Autodesk Fusion 360 part; units mm, degrees
sketch "Esquisse1" plane through (0, 0, 0) normal (0, 0, 1) x (1, 0, 0)
  line L0 (0, 0) -> (66, 0) construction
  line L1 (66, 53) -> (0, 53) construction
  line L2 (0, 53) -> (0, 0) construction
  line L3 (66, 0) -> (66, 2) construction
  line L4 (66, 2) -> (69, 5) construction
  line L5 (69, 5) -> (69, 37) construction
  line L6 (69, 37) -> (66, 40) construction
  line L7 (66, 40) -> (66, 53) construction
  line L8 (-0.2, -0.2) -> (66.2, -0.2)
  line L9 (66.2, -0.2) -> (66.2, 1.9172)
  line L10 (66.2, 1.9172) -> (69.2, 4.9172)
  line L11 (69.2, 4.9172) -> (69.2, 37.0828)
  line L12 (69.2, 37.0828) -> (66.2, 40.0828)
  line L13 (66.2, 40.0828) -> (66.2, 53.2)
  line L14 (66.2, 53.2) -> (-0.2, 53.2)
  line L15 (-0.2, 53.2) -> (-0.2, -0.2)
  dimension "d1" = 66
  dimension "d2" = 53
  dimension "d6" = 37
  dimension "d7" = 40
  dimension "d10" = 3
  dimension "d11" = 3
  dimension "d12" = 2
  dimension "d24" = 0.2
sketch "Esquisse2" plane through (0, 0, 0) normal (0, 0, 1) x (1, 0, 0)
  circle A0 centre (14.1, 2.5) radius 1
  circle A1 centre (66.5, 35) radius 1
  circle A2 centre (66.5, 7) radius 1
  line L0 (0, 53) -> (0, 0)
  line L1 (66, 53) -> (0, 53)
  line L2 (69, 5) -> (69, 37)
  line L3 (66.5, 7) -> (66.5, 35) construction
  line L4 (0, 0) -> (66, 0) construction
  circle A3 centre (14.1, 2.5) radius 2.7
  circle A4 centre (66.5, 35) radius 2.7
  circle A5 centre (66.5, 7) radius 2.7
  line L5 (69.2, 37.0828) -> (66.2, 40.0828)
  line L6 (66.2, 40.0828) -> (66.2, 53.2)
  line L7 (66.2, 40.0828) -> (64.1305, 36.2944)
  line L8 (69.2, 4.9172) -> (69.2, 37.0828)
  line L9 (66.5, 32.3) -> (69.2, 32.3)
  arc A6 (64.1305, 36.2944) -> (66.5, 32.3) centre (66.5, 35) ccw
  line L10 (66.2, 1.9172) -> (69.2, 4.9172)
  line L11 (66.2, -0.2) -> (66.2, 1.9172)
  line L12 (66.2, 1.9172) -> (64.1305, 5.7056)
  line L13 (66.5, 9.7) -> (69.2, 9.7)
  arc A7 (66.5, 9.7) -> (64.1305, 5.7056) centre (66.5, 7) ccw
  line L14 (-0.2, -0.2) -> (66.2, -0.2)
  line L15 (16.8, 2.5) -> (16.8, -0.2)
  line L16 (11.4, 2.5) -> (11.4, -0.2)
  arc A8 (16.8, 2.5) -> (11.4, 2.5) centre (14.1, 2.5) ccw
  line L17 (0, 48) -> (10, 48)
  line L18 (10, 48) -> (10, 53) construction
  arc A9 (10, 48) -> (15, 53) centre (10, 53) ccw
  dimension "d14" = 2
  dimension "d15" = 2
  dimension "d16" = 2
  dimension "d17" = 14.1
  dimension "d20" = 2.5
  dimension "d21" = 7
  dimension "d22" = 2
  dimension "d33" = 1.7
  dimension "d34" = 2.5
  dimension "d45" = 5
  dimension "d46" = 10
  dimension "d85" = 2.7
sketch "Esquisse3" plane through (0, 0, 0) normal (0, 0, 1) x (1, 0, 0)
  line L0 (-4, -1.7) -> (70.7, -1.7)
  line L1 (70.7, -1.7) -> (70.7, 54.7)
  line L2 (70.7, 54.7) -> (-4, 54.7)
  line L3 (-4, 54.7) -> (-4, -1.7)
  line L4 (-0.2, -0.2) -> (66.2, -0.2)
  line L5 (69.2, 4.9172) -> (69.2, 37.0828)
  line L6 (-5, -2.7) -> (71.7, -2.7)
  line L7 (71.7, -2.7) -> (71.7, 55.7)
  line L8 (71.7, 55.7) -> (-5, 55.7)
  line L9 (-5, 55.7) -> (-5, -2.7)
  dimension "d26" = 56.4
  dimension "d27" = 1.5
  dimension "d28" = 74.7
  dimension "d29" = 1.5
  dimension "d52" = 1
extrude "Extrusion1" add sketch "Esquisse3" against normal blind 1.5 contours L0 L1 L2 L3
sketch "Esquisse4" plane through (0, 0, 0) normal (0, 0, 1) x (-1, 0, 0)
  line L0 (4, -54.7) -> (4, 1.7)
  line L1 (4, 1.7) -> (-70.7, 1.7)
  line L2 (-70.7, 1.7) -> (-70.7, -54.7)
  line L3 (-70.7, -54.7) -> (4, -54.7)
  line L4 (4, -54.7) -> (-70.7, -54.7)
  line L5 (-70.7, -54.7) -> (-70.7, 1.7)
  line L6 (-70.7, 1.7) -> (4, 1.7)
  line L7 (4, 1.7) -> (4, -54.7)
  line L8 (2.5, -53.2) -> (-69.2, -53.2)
  line L9 (-69.2, -53.2) -> (-69.2, 0.2)
  line L10 (-69.2, 0.2) -> (2.5, 0.2)
  line L11 (2.5, 0.2) -> (2.5, -53.2)
  line L12 (-66.2, 0.2) -> (-66.2, -1.9172)
  line L13 (-66.2, -1.9172) -> (-69.2, -4.9172)
  line L14 (-66.2, -40.0828) -> (-66.2, -53.2)
  line L15 (-69.2, -37.0828) -> (-66.2, -40.0828)
  line L16 (0.2, -53.2) -> (0.2, 0.2)
  dimension "d32" = 1.5
extrude "Extrusion2" add sketch "Esquisse2" along normal blind 2 contours L2 A5 A7 | L2 A4 A6 | A3 A8
extrude "Extrusion3" cut 3 faces at (16.2233, 2.6341, 2) (68.5, 7, 2) (68.5, 35, 2) along direction (0, 0, -1) blind 2
extrude "Extrusion4" add sketch "Esquisse2" sketch "Esquisse4" along normal blind 3 contours L2 A5 A7 | A5 L8 L10 L12 | L2 A5 | L2 A5 L13 | L2 A5 L8 L13 | A3 L14 L15 | L2 A4 L9 | L2 A4 L8 L9 | L2 A4 A6 | L2 A4 | A4 L5 L7 L8 | A3 L14 L16 | A3 A8 of sketch 2 contours L8 L9 L14 L15 | L9 L10 L12 L13
extrude "Extrusion5" add sketch "Esquisse4" along normal blind 4.5 contours L8 L10 L11 L16
extrude "Extrusion6" add sketch "Esquisse3" sketch "Esquisse4" along normal blind 20.4 and the other way up to surface of sketch 2 second end surface through (0, 0, -1.5) normal (0, 0, -1) offset 0
extrude "Extrusion7" add sketch "Esquisse2" along normal blind 3 contours L0 L1 L17 A9
sketch "Esquisse5" plane through (0, 0, -1.5) normal (0, 0, -1) x (1, 0, 0)
  line L0 (70.7, -26.5) -> (-4, -26.5) construction
  circle A0 centre (45.8, -26.5) radius 1.5
  circle A1 centre (20.9, -26.5) radius 1.5
  line L1 (20.9, -28) -> (-4, -28) construction
  line L2 (20.9, -28) -> (45.8, -28) construction
  line L3 (45.8, -28) -> (70.7, -28) construction
  line L4 (71.7, 2.7) -> (-5, 2.7)
  line L5 (-5, 2.7) -> (-5, -55.7)
  line L6 (-5, -55.7) -> (71.7, -55.7)
  line L7 (71.7, -55.7) -> (71.7, 2.7)
  dimension "d49" = 3
extrude "Extrusion8" cut sketch "Esquisse5" against normal blind 1.5 contours A0 | A1
extrude "Extrusion11" add 1 faces at (-2.5, 17.6, 9.8) along direction (1, 0, 0) blind 1
extrude "Extrusion12" cut 1 faces at (-5, 36.2333, 5.8) along direction (1, 0, 0) blind 1
sketch "Esquisse10" plane through (-1.5, 0, 0) normal (1, 0, 0) x (0, 1, 0)
  line L0 (-0.2, 4.5) -> (53.2, 4.5)
  line L1 (53.2, 4.5) -> (53.2, 20.4)
  line L2 (53.2, 20.4) -> (-0.2, 20.4)
  line L3 (-0.2, 20.4) -> (-0.2, 4.5)
  line L4 (-1.2, 18.9) -> (54.2, 18.9)
  line L5 (54.2, 18.9) -> (54.2, 15.7)
  line L6 (54.2, 15.7) -> (-1.2, 15.7)
  line L7 (-1.2, 15.7) -> (-1.2, 18.9)
  line L8 (26.5, 18.9) -> (26.5, 20.4) construction
  line L9 (-0.2, 18.9) -> (-0.2, 20.4)
  line L10 (-0.2, 20.4) -> (53.2, 20.4)
  dimension "d89" = 1.5
  dimension "d90" = 3.2
  dimension "d93" = 55.4
extrude "Extrusion17" cut sketch "Esquisse10" against normal up to surface (2.5 mm away) contours L3 L4 L6 L7 | L1 L3 L4 L6 | L1 L4 L5 L6 | L1 L2 L3 L4 L9 L10
extrude "Extrusion18" cut sketch "Esquisse10" along normal blind 71.5 contours L3 L4 L6 L7 | L1 L3 L4 L6 | L1 L4 L5 L6
sketch "Esquisse11" plane through (0, 0, 15.7) normal (0, 0, 1) x (-1, 0, 0)
  line L0 (-70, -54.2) -> (4, -54.2)
  line L1 (4, -54.2) -> (4, 1.2)
  line L2 (4, 1.2) -> (-70, 1.2)
  line L3 (-70, 1.2) -> (-70, -54.2)
  line L4 (1.5, -53.2) -> (-69.2, -53.2)
  line L5 (-69.2, -53.2) -> (-69.2, 0.2)
  line L6 (-69.2, 0.2) -> (1.5, 0.2)
  line L7 (1.5, 0.2) -> (1.5, -53.2)
  line L8 (1.9, -54.2) -> (1.9, 1.2)
  dimension "d98" = 71.9
extrude "Extrusion19" add sketch "Esquisse11" along normal blind 0.2 contours L0 L1 L2 L8
sketch "Esquisse7" plane through (-1.5, 0, 0) normal (1, 0, 0) x (0, 1, 0)
  line L0 (-0.2, 15.7) -> (-0.2, 4.5)
  line L1 (-0.2, 4.5) -> (53.2, 4.5)
  line L2 (53.2, 4.5) -> (53.2, 15.7)
  line L3 (3.8, 4.5) -> (13.2, 4.5)
  line L4 (13.2, 4.5) -> (13.2, 15.9)
  line L5 (13.2, 15.9) -> (3.8, 15.9)
  line L6 (3.8, 15.9) -> (3.8, 4.5)
  line L7 (33.4, 4.5) -> (41.8, 4.5)
  line L8 (41.8, 4.5) -> (41.8, 7.7)
  line L9 (41.8, 7.7) -> (33.4, 7.7)
  line L10 (33.4, 7.7) -> (33.4, 4.5)
  line L11 (53.2, 15.7) -> (-0.2, 15.7)
  dimension "d66" = 9.4
  dimension "d67" = 11.4
  dimension "d68" = 4
  dimension "d71" = 8.4
  dimension "d72" = 3.2
  dimension "d73" = 11.4
extrude "Extrusion14" cut sketch "Esquisse7" against normal blind 2.5 contours L1 L3 L4 L6 L11 | L4 L5 L6 L11 | L1 L7 L8 L9 L10
sketch "Esquisse8" plane through (-4, 0, 0) normal (-1, 0, 0) x (0, -1, 0)
  line L0 (-3.8, 4.5) -> (-13.2, 4.5)
  line L1 (-13.2, 4.5) -> (-13.2, 15.9)
  line L2 (-3.8, 15.9) -> (-3.8, 4.5)
  line L3 (-33.4, 4.5) -> (-41.8, 4.5)
  line L4 (-41.8, 4.5) -> (-41.8, 7.7)
  line L5 (-41.8, 7.7) -> (-33.4, 7.7)
  line L6 (-33.4, 7.7) -> (-33.4, 4.5)
  line L7 (-53.2, 20.4) -> (-55.7, 20.4)
  line L8 (-55.7, -1.5) -> (2.7, -1.5)
  line L9 (-31.9, 3) -> (-43.3, 3)
  line L10 (-43.3, 3) -> (-43.3, 9.2)
  line L11 (-43.3, 9.2) -> (-31.9, 9.2)
  line L12 (-31.9, 9.2) -> (-31.9, 3)
  line L13 (2.7, -1.5) -> (2.7, 20.4)
  line L14 (-55.7, 20.4) -> (-55.7, -1.5)
  line L15 (-13.2, 15.9) -> (-54.2, 15.9)
  line L16 (-54.2, 15.9) -> (-54.2, 18.9)
  line L17 (-54.2, 18.9) -> (-53.2, 18.9)
  line L18 (-53.2, 18.9) -> (-53.2, 20.4)
  line L19 (2.7, 20.4) -> (0.2, 20.4)
  line L20 (0.2, 20.4) -> (0.2, 18.9)
  line L21 (0.2, 18.9) -> (1.2, 18.9)
  line L22 (1.2, 18.9) -> (1.2, 15.9)
  line L23 (1.2, 15.9) -> (-3.8, 15.9)
  dimension "d79" = -1.5
extrude "Extrusion16" cut sketch "Esquisse8" against normal blind 1.5 contours L9 L10 L11 L12
chamfer "Chanfrein1" distance 1.5 angle 45 4 edges at (-4, 31.9, 6.1) (-4, 37.6, 9.2) (-4, 43.3, 6.1) (-4, 37.6, 3)
draft "Dépouille1" angle 0.2 neutral plane through (70, 0, 0) pull (-1, 0, 0) 1 faces at (45.0667, -0.8667, 18.9)
equation "d1 = longArduino"
equation "d2 = largArduino"
equation "longArduino = 66 mm"
equation "largArduino = 53 mm"
equation "d6 = longEncoche - largEncoche"
equation "d7 = longEncoche"
equation "longEncoche = 40 mm"
equation "largEncoche = 3 mm"
equation "d10 = largEncoche"
equation "d11 = largEncoche"
equation "percageArduino = 2 mm"
equation "d14 = percageArduino"
equation "d15 = percageArduino"
equation "d16 = percageArduino"
equation "decalagePercage = 2.5 mm"
equation "d20 = decalagePercage"
equation "decalageImpression = 0.2 mm"
equation "d24 = decalageImpression"
equation "epaisseurBoitier = 1.5 mm"
equation "d26 = largArduino + ( epaisseurBoitier + decalageImpression ) * 2"
equation "d27 = epaisseurBoitier"
equation "d28 = longArduino + largEncoche + epaisseurBoitier + decalageImpression + 4 mm"
equation "d29 = epaisseurBoitier"
equation "d33 = epaisseurBoitier + decalageImpression"
equation "d34 = decalagePercage"
equation "d41 = 3 mm + 1.5 mm"
equation "d43 = 20 mm - 1.3 mm + epaisseurBoitier + decalageImpression"
equation "largPriseDC = 9 mm"
equation "longPriseDC = 11 mm"
equation "d66 = largPriseDC + decalageImpression * 2"
equation "d67 = longPriseDC + decalageImpression * 2"
equation "largPriseUSB = 3 mm"
equation "longPriseUSB = 8 mm"
equation "d71 = longPriseUSB + decalageImpression * 2"
equation "d72 = largPriseUSB + decalageImpression"
equation "epaisseurPlexi = 3 mm"
equation "d89 = epaisseurBoitier"
equation "d90 = epaisseurPlexi + decalageImpression"
equation "largeurPlexi = 55 mm"
equation "longueurPlexi = 71.5 mm"
equation "d93 = largeurPlexi + decalageImpression * 2"
equation "d96 = longueurPlexi"
equation "d98 = longueurPlexi + decalageImpression * 2"
equation "d99 = decalageImpression"
Geometry: final body of the model. Coordinates: model frame, mm. A direction names the side the tool comes from. Round coordinates to 2 decimals unless told otherwise and drop trailing zeros. Order: outer loops, then holes, each group sorted by start corner. A loop starts at its lowest first (then second) coordinate and runs counter-clockwise, first axis right, second up. Notation, with made-up numbers: M 12.5,78.25 L 32.5,78.25 A25 ccw 32.5,101.25 Z; hole C 80.5,60 d11. An arc over 180 degrees is marked long. Use one line per item in the form item = value. Start each with the question number.
Q1. Mould query, pull axis Z, two halves, no side actions, for faces 4 (the face through (-3.2, 37.5, 2.3)), 5 (the face through (7, 51, 3)), 6 (the face through (65.763, 34.324, 1.479)). Classes: +Z half, -Z half, draft (parallel to the pull), parting line (faces both ways), or undercut.
Q2. Material intervals for line 1 (X direction, y = 26.5, z = -0.7); line 2 (Y direction, x = 66.5, z = 1.6); line 3 (Y direction, x = 45.8, z = -0.7), sorted ascending. Write a range as [from, to].
Q3. Access query for faces 1 (the face through (66.2, 1, 1)), 2 (the face through (-3.2, 37.7, 9.9)), 3 (the face through (70, 26, 20.4)). Directions: +Z, -Z, +X, -X, +Y, -Y. A direction counts if a zero-diameter tool reaches every point of the face in a straight line with its end or side. Return the directions, or none.
Q4. Cut plane A-A (y = 26.5). Return loops of the section in (x, z).
Q5. Cut plane B-B (x = 20.9). Return loops of the section in (y, z), and give its area (3 significant figures).
Q6. Pin query (flat end, axial travel): pin 1 Ø2.5 at (x, y) = (20.9, 26.5) entering from -Z; pin 2 Ø0.6 at (x, y) = (-3, 0.5) entering from +Z; pin 3 Ø1.5 at (x, y) = (24, 43) entering from +Z. Return the tip coordinate at first contact, or that it passes through.
Q7. Cut plane D-D (x = 4.5). Return loops of the section in (y, z).
Q8. Cut plane C-C (z = 12.75). Return loops of the section in (x, y).
Geometry results:
q1.face_4 = undercut
q1.face_5 = +Z half
q1.face_6 = draft
q2.line_1 = [-4, 19.4], [22.4, 44.3], [47.3, 71.7]
q2.line_2 = [-2.7, 6], [8, 9.7], [32.3, 34], [36, 55.7]
q2.line_3 = [-2.7, 25], [28, 55.7]
q3.face_1 = +Z
q3.face_2 = -X
q3.face_3 = +Z, +X, -X, +Y, -Y
q4.outline = M -4,-1.5 L 19.4,-1.5 L 19.4,0 L -0.2,0 L -0.2,4.5 L -1.5,4.5 L -1.5,15.7 L -1.9,15.7 L -1.9,15.9 L -4,15.9 Z; M 22.4,-1.5 L 44.3,-1.5 L 44.3,0 L 22.4,0 Z; M 47.3,-1.5 L 71.7,-1.5 L 71.7,20.4 L 69.2,20.4 L 69.2,18.9 L 70,18.9 L 70,15.7 L 69.2,15.7 L 69.2,0 L 47.3,0 Z
q5.outline = M -2.7,-1.5 L 25,-1.5 L 25,0 L -0.2,0 L -0.2,15.7 L -1.2,15.7 L -1.2,19.07 L -0.2,19.07 L -0.2,20.4 L -2.7,20.4 Z; M 28,-1.5 L 55.7,-1.5 L 55.7,20.4 L 53.2,20.4 L 53.2,19.07 L 54.2,19.07 L 54.2,15.7 L 53.2,15.7 L 53.2,0 L 28,0 Z
q5.area = 178 mm^2
q6.pin_1 = through
q6.pin_2 = 15.9
q6.pin_3 = 0
q7.outline = M -2.7,-1.5 L 55.7,-1.5 L 55.7,20.4 L 53.2,20.4 L 53.2,19.13 L 54.2,19.13 L 54.2,15.7 L 53.2,15.7 L 53.2,0 L 53,0 L 53,3 L 48,3 L 48,0 L -0.2,0 L -0.2,15.7 L -1.2,15.7 L -1.2,19.13 L -0.2,19.13 L -0.2,20.4 L -2.7,20.4 Z
q8.outline = M -4,-2.7 L 71.7,-2.7 L 71.7,55.7 L -4,55.7 L -4,13.2 L -1.5,13.2 L -1.5,53.2 L 69.2,53.2 L 69.2,-0.2 L -1.5,-0.2 L -1.5,3.8 L -4,3.8 Z
